```python
from build123d import *

# Parameters (mm, degrees)
F1_DEPTH = 508
F2_W     = 1436.565518
F2_H     = 80.049575
F2_W_2   = 1436.565519
F2_H_2   = 90.867102
F2_W_3   = 1440.892518
F2_H_3   = 73.559083
F3_DEPTH = 254


with BuildPart() as f1:
    # F0 (on Front) → F1 (new body)
    with BuildSketch(Plane.XZ):
        Polygon((759.084124, 116.439129), (-773.183558, 116.439129), (-764.915876, -24.110599), (759.084124, -24.110599), align=None)
    extrude(amount=F1_DEPTH)

    # F2 (on face) → F3 (cut)
    with BuildSketch(Plane.XY.offset(116.439129)):
        with Locations((-18.949032, -415.180921)):
            Rectangle(F2_W, F2_H)
        with Locations((-16.785503, -249.673009)):
            Rectangle(F2_W_2, F2_H_2)
        with Locations((-14.622003, -106.881854)):
            Rectangle(F2_W_3, F2_H_3)
    extrude(amount=-F3_DEPTH, mode=Mode.SUBTRACT)


solid = f1.part
```
Build history of the part. All positions in model axes, mm. A direction names the side the tool comes from. Give positions to 0.01 mm unless a question says otherwise; leave off trailing zeros. Loops run counter-clockwise (first coordinate to the right, second up) from the corner with the lowest first, then second, coordinate; pieces in that order, holes last. Notation, with made-up numbers: (64, 69.25) -> (102, 69.25) arc R15 ccw to (102, 98.25) -> close; hole circle Ø10 at (76.5, 79). An arc over 180 degrees is marked (long way). One line per question, with ' | ' between items.
Q1. Cut at A-A, the plane y = -120. Write the cut outline in (x, z).
Filled sheet:
outline: (-773.18, 116.44) -> (-764.92, -24.11) -> (-735.07, -24.11) -> (-735.07, 116.44) -> close; (705.82, -24.11) -> (759.08, -24.11) -> (759.08, 116.44) -> (705.82, 116.44) -> close
Q2. Cut at B-B, the plane x = -301. Write the cut outline in (y, z), plus the area to 3 significant figures.
Filled sheet:
outline: (-508, -24.11) -> (-455.21, -24.11) -> (-455.21, 116.44) -> (-508, 116.44) -> close; (-375.16, -24.11) -> (-295.11, -24.11) -> (-295.11, 116.44) -> (-375.16, 116.44) -> close; (-204.24, -24.11) -> (-143.66, -24.11) -> (-143.66, 116.44) -> (-204.24, 116.44) -> close; (-70.1, -24.11) -> (0, -24.11) -> (0, 116.44) -> (-70.1, 116.44) -> close | area: 37,000 mm²
Q3. Tool access for faces 1 (the flat face through (-27, -204.239, 47)), 2 (the flat face through (-14, -307, -24.111)): list every direction of +Z, -Z, +X, -X, +Y, -Y with a clear straight run to the whole face (end or side of a thin tool).
Filled sheet:
face 1: +Z, -Z | face 2: -Z, +X, -X, +Y, -Y
Q4. Pull direction X, two halves, no side cores. Call faces 3 (the flat face through (4, -307, 116.439)), 4 (the flat face through (-769.108, -250.444, 47.148)), 5 (the flat face through (-735.068, -250, 47)): pulls with the +X half, pulls with the -X half, needs draft (parallel to the pull), parting line crosses it, or undercut.
Filled sheet:
face 3: needs draft | face 4: pulls with the -X half | face 5: undercut
Q5. Drill centre lines: line 1 along Y through (x, z) = (437, 59); line 2 along X through (y, z) = (-213.5, 45); line 3 along X through (y, z) = (-395.5, 67). Where is each one in solid material? Low to high. Write a range as [from, to].
Filled sheet:
line 1: y = [-508, -455.21], [-375.16, -295.11], [-204.24, -143.66], [-70.1, 0] | line 2: x = [-768.98, -735.07], [701.5, 759.08] | line 3: x = [-770.28, -737.23], [699.33, 759.08]
Q6. Drop a flat-ended pin along its axis: pin 1 (1.5 mm diameter, centred on x = -411, z = 97.5, fed in from +Y). Give the stop position or say it passes through.
Filled sheet:
pin 1: stops at y = 0
Q7. Cut at C-C, the plane z = 45. Write the cut outline in (x, y).
Filled sheet:
outline: (-768.98, -508) -> (759.08, -508) -> (759.08, 0) -> (-768.98, 0) -> close; hole (-737.23, -455.21) -> (699.33, -455.21) -> (699.33, -375.16) -> (-737.23, -375.16) -> close; hole (-735.07, -295.11) -> (701.5, -295.11) -> (701.5, -204.24) -> (-735.07, -204.24) -> close; hole (-735.07, -143.66) -> (705.82, -143.66) -> (705.82, -70.1) -> (-735.07, -70.1) -> close
